Input: part model. Units: mm. Frame: model coordinates. A direction names the side the tool comes from. Coordinates: 2 decimals unless noted, no trailing zeros. Loops run counter-clockwise (first coordinate to the right, second up) from the corner with the lowest first, then second, coordinate; pieces in that order, holes last. Notation, with made-up numbers: (-13, 78) - (16, 78) arc R31 ccw to (16, 115) - close; hole circle Ø8 at (36, 24). An arc over 180 degrees is marked (long way). Use a Markdown table: item, result. Add a question column.
1. Section query C-C on x = -14. Return the cut outline in (y, z) (3 decimals), then the cut area to 3 significant figures.
2. Draft query along X for faces 1 (the face through (33.574, 10.437, -4.775)), 2 (the face through (32.33, 1.01, -24)), 3 (the face through (0, 0, 0)). Return one class per face: released by +X, released by -X, zero draft, split by the parting line, or undercut.
3. Section query D-D on z = 10. Return the cut outline in (x, y), then the cut area to 3 significant figures.
4. Access query for faces 4 (the face through (11.56, 4, 24)), 5 (the face through (-25.56, 4, 24)), 6 (the face through (-19, 4, 28.845)), 7 (the face through (-19, 4, 18.845)), 8 (the face through (24.56, 4, -5)). Directions: +Z, -Z, +X, -X, +Y, -Y. A direction counts if a zero-diameter tool reaches every point of the face in a straight line with its end or side. Return the directions, or none.
5. Ray query, L1, parallel to Z at x = -30.48, y = 0.75 (3 decimals); L2, parallel to Y at x = -10.5, z = 25.5; L3, parallel to Z at x = 23, y = 3.25 (3 decimals). Return the intervals inside material, ascending. Write a range as [from, to].
6. Section query A-A on x = -30.48. Return the cut outline in (y, z) (3 decimals).
7. Contact query for flat-ended pins moving along their axis: P1, Ø3, axis at x = 1.5, z = -3.5, coming from the +Y side; P2, Ø3, axis at x = 19, y = 6.5, coming from the -Z side (3 decimals); P3, Ø3, axis at x = 26, z = 16.5, coming from the -Y side; P4, Ø8, axis at x = -17, z = 26, coming from the +Y side. Output: stop coordinate, or through.
8. Section query B-B on y = 4.5. Return the cut outline in (x, z) (3 decimals).
```python
from build123d import *

# Parameters (mm, degrees)
SKETCH1_W           = 71.12
SKETCH1_H           = 59.69
BOSS_EXTRUDE1_DEPTH = 2
SKETCH2_R           = 2
CUT_EXTRUDE1_DEPTH  = 2
SKETCH3_W           = 14
SKETCH3_H           = 10
BOSS_EXTRUDE2_DEPTH = 5
SKETCH4_W           = 10
SKETCH4_H           = 10
BOSS_EXTRUDE3_DEPTH = 13
CUT_EXTRUDE2_DEPTH  = 31


with BuildPart() as part:
    # Sketch1 → Boss-Extrude1 (new body)
    with BuildSketch(Plane(origin=(0, 0, 0), x_dir=(1, 0, 0), z_dir=(0, 1, 0))):
        Rectangle(SKETCH1_W, SKETCH1_H)
    extrude(amount=BOSS_EXTRUDE1_DEPTH)

    # Sketch2 → Cut-Extrude1 (cut)
    with BuildSketch(Plane(origin=(0, 2, 0), x_dir=(1, 0, 0), z_dir=(0, 1, 0))):
        with Locations((-30.48, 24.765)):
            Circle(SKETCH2_R)
        with Locations((30.48, 24.765)):
            Circle(SKETCH2_R)
        with Locations((30.48, -24.765)):
            Circle(SKETCH2_R)
        with Locations((-30.48, -24.765)):
            Circle(SKETCH2_R)
    extrude(amount=-CUT_EXTRUDE1_DEPTH, mode=Mode.SUBTRACT)

    # Sketch3 → Boss-Extrude2 (add)
    with BuildSketch(Plane(origin=(0, 2, 0), x_dir=(1, 0, 0), z_dir=(0, 1, 0))):
        with Locations((-18.56, -23.845)):
            Rectangle(SKETCH3_W, SKETCH3_H)
        with Locations((18.56, -23.845)):
            Rectangle(SKETCH3_W, SKETCH3_H)
    extrude(amount=BOSS_EXTRUDE2_DEPTH)

    # Sketch4 → Boss-Extrude3 (add)
    with BuildSketch(Plane(origin=(0, 2, 0), x_dir=(1, 0, 0), z_dir=(0, 1, 0))):
        with Locations((29.56, 4.845)):
            Rectangle(SKETCH4_W, SKETCH4_H)
    extrude(amount=BOSS_EXTRUDE3_DEPTH)

    # Sketch7 → Cut-Extrude2 (cut, through all)
    with BuildSketch(Plane.XY.offset(0.155)):
        Polygon((26.56, 15), (24.56, 6), (24.56, 15), align=None)
        Polygon((34.56, 6), (32.56, 15), (34.56, 15), align=None)
    extrude(amount=-CUT_EXTRUDE2_DEPTH, mode=Mode.SUBTRACT)


solid = part.part
```
Resolved:
| question | item | result |
|---|---|---|
| 1 | outline | (0, -29.845) - (2, -29.845) - (2, 18.845) - (7, 18.845) - (7, 28.845) - (2, 28.845) - (2, 29.845) - (0, 29.845) - close |
| 1 | area | 169 mm² |
| 2 | face 1 | released by +X |
| 2 | face 2 | undercut |
| 2 | face 3 | zero draft |
| 3 | outline | (-35.56, 0) - (35.56, 0) - (35.56, 2) - (-35.56, 2) - close |
| 3 | area | 142 mm² |
| 4 | face 4 | +Z, -Z, +Y |
| 4 | face 5 | +Z, -Z, -X, +Y |
| 4 | face 6 | +Z, +X, -X, +Y |
| 4 | face 7 | -Z, +X, -X, +Y |
| 4 | face 8 | -Z, -X, +Y |
| 5 | L1 | [-29.845, -26.765], [-22.765, 22.765], [26.765, 29.845] |
| 5 | L2 | [0, 2] |
| 5 | L3 | [18.845, 28.845] |
| 6 | outline | (0, -29.845) - (2, -29.845) - (2, -26.765) - (0, -26.765) - close; (0, -22.765) - (2, -22.765) - (2, 22.765) - (0, 22.765) - close; (0, 26.765) - (2, 26.765) - (2, 29.845) - (0, 29.845) - close |
| 7 | P1 | y = 2 |
| 7 | P2 | z = 18.845 |
| 7 | P3 | y = 0 |
| 7 | P4 | y = 7 |
| 8 | outline | (-25.56, 18.845) - (-11.56, 18.845) - (-11.56, 28.845) - (-25.56, 28.845) - close; (11.56, 18.845) - (25.56, 18.845) - (25.56, 28.845) - (11.56, 28.845) - close; (24.56, -9.845) - (34.56, -9.845) - (34.56, 0.155) - (24.56, 0.155) - close |
